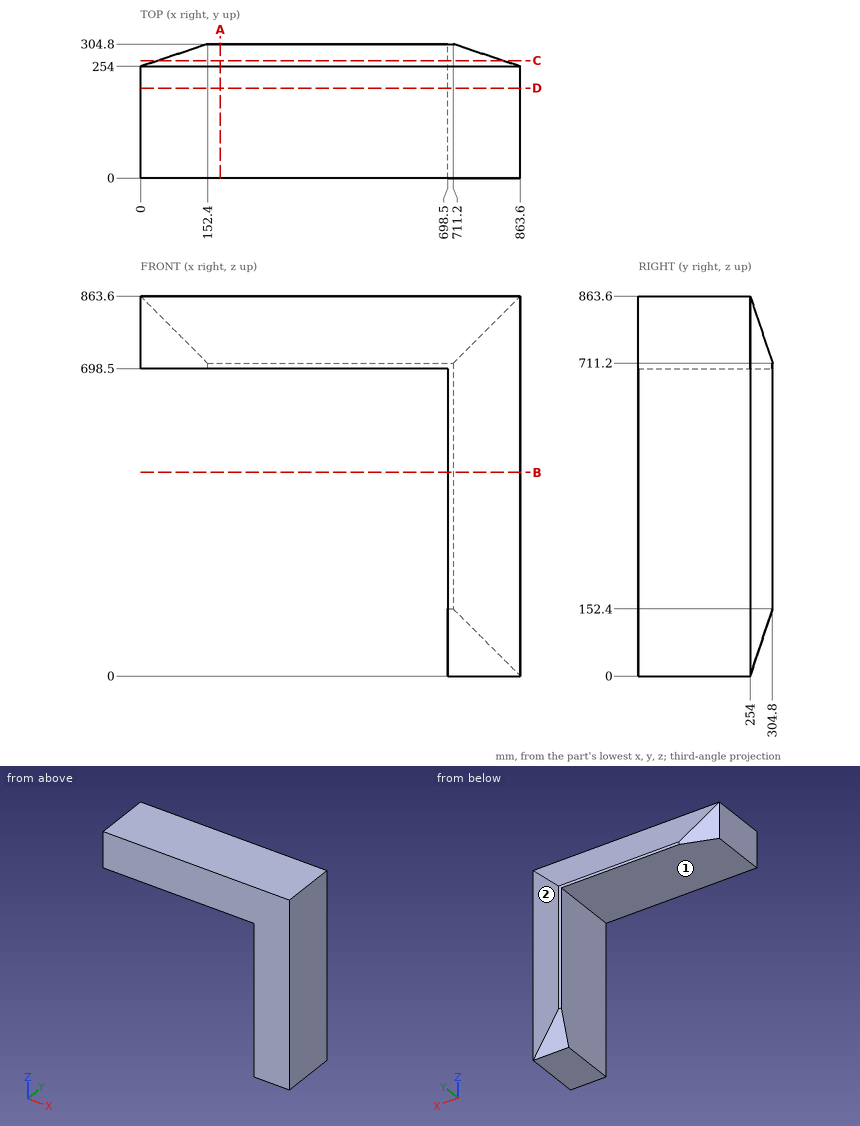
Job drawing, mm, ordinate dimensions from the low corner. One solid piece. A direction names the side the tool comes from. Give positions to 0.01 mm unless a question says otherwise; leave off trailing zeros. Order: outer loops, then holes, each group sorted by start corner. A loop starts at its lowest first (then second) coordinate and runs counter-clockwise, first axis right, second up. Notation, with made-up numbers: M 44,34.25 L 55,34.25 A19 cw 55,66.25 Z; hole C -11.5,-16 d7. An arc over 180 degrees is marked long. Return JSON: item names as keys, results as strings.
Q1. 3-axis set-ups, long thin cutter, end or side, ignore diameter. For the marked faces 1 and 2: which of +Z, -Z, +X, -X, +Y, -Y reach the whole face in a straight line?
Answer list:
{"face 1": "-Z, -X, +Y, -Y", "face 2": "+Z, -Z, +X, +Y"}
Q2. Flat gauge pins, fed straight in: pin 1 (8 mm diameter, centred on y = 34, z = 164.5, fed in from -X); pin 2 (8 mm diameter, centred on x = 676.5, y = 245.5, fed in from -Z). Where does each tip first touch, or does it go through?
Answer list:
{"pin 1": "stops at x = 698.5", "pin 2": "stops at z = 698.5"}
Q3. Band-saw the part on D-D (y = 204.5). Give the cut face in (x, z).
Answer list:
{"outline": "M 0,698.5 L 698.5,698.5 L 698.5,0 L 863.6,0 L 863.6,863.6 L 0,863.6 Z"}
Q4. Band-saw the part on A-A (x = 181.5). Give the cut face in (y, z), then the cut area to 3 significant figures.
Answer list:
{"outline": "M 0,698.5 L 304.8,698.5 L 304.8,711.2 L 254,863.6 L 0,863.6 Z", "area": "46,500 mm^2"}
Q5. Band-saw the part on B-B (z = 463). Give the cut face in (x, y).
Answer list:
{"outline": "M 698.5,0 L 863.6,0 L 863.6,254 L 711.2,304.8 L 698.5,304.8 Z"}
Q6. Wall check: probe 1 along X at (y, z) = (242.5, 582.5); probe 2 along Y at (x, z) = (747.5, 462). Give the ranges that are in metal, low to high. Write a range as from..to.
Answer list:
{"probe 1": "x = 698.5..863.6", "probe 2": "y = 0..292.7"}
Q7. Band-saw the part on C-C (y = 267). Give the cut face in (x, z).
Answer list:
{"outline": "M 39,698.5 L 698.5,698.5 L 698.5,39 L 824.6,39 L 824.6,824.6 L 39,824.6 Z"}
